Geometry check sheet. Reference: drawing and pictorial views, mm from the part's lowest x, y, z. A direction names the side the tool comes from. Give positions to 0.01 mm unless a question says otherwise; leave off trailing zeros. Write each loop counter-clockwise with the first axis right and the second up, starting at its lowest first coordinate (ties: lowest second). Pieces come first, ordered by that corner, then holes. Notation, with made-up numbers: M 78.5,52.5 L 96.5,52.5 A14 cw 96.5,72.5 Z; hole C -34,10.5 d7. An arc over 180 degrees is marked long. Write item = value, one per line. Start each with the question number.
1) Cross-section at B-B, the plane z = 29.5. Record the cut outline in (x, y).
2) Scan lines: line 1 along X through (y, z) = (6.25, 6); line 2 along Y through (x, z) = (37, 29.1); line 3 along Z through (x, y) = (20, 4.75). Record each from-to range of solid material in increasing order. Write a range as [from, to].
3) Cross-section at C-C, the plane y = 12.5. Record the cut outline in (x, z).
4) Cross-section at D-D, the plane z = 6. Record the cut outline in (x, y), plus the area to 3 significant figures.
5) Mould release check, pull along Z, two halves, no side actions. Record for the marked faces 1, 2, 3 and 4: released by +Z, released by -Z, zero draft, split by the parting line, or undercut.
6) Go/stop test with flat-tipped pins: pin 1 (2.5 mm diameter, centred on y = 5.5, z = 28.5, fed in from -X); pin 2 (10.5 mm diameter, centred on x = 7, y = 11, fed in from -Z); pin 3 (1.2 mm diameter, centred on x = 5.5, z = 29, fed in from -Y); pin 4 (12 mm diameter, centred on y = 5.5, z = 25.5, fed in from +X). Record where each tip stops, or that it passes through.
7) Cross-section at A-A, the plane y = 3.5. Record the cut outline in (x, z), plus the area to 3 significant figures.
8) Access from +Z, -Z, +X, -X, +Y, -Y to the whole of each face (thin tool, end or side, straight path). Record for the marked faces 5, 6, 7, 8 and 9.
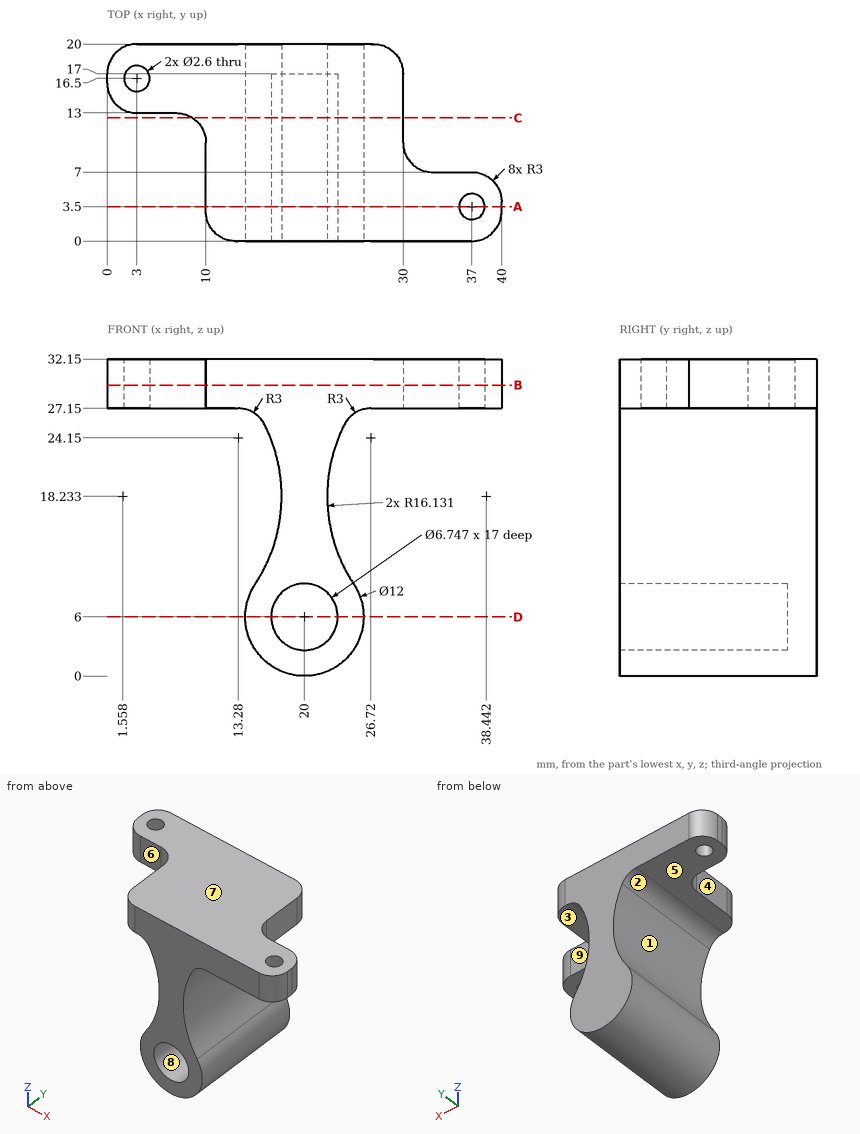
Reply:
q1.outline = M 0,16 A3 ccw 3,13 L 7,13 A3 cw 10,10 L 10,3 A3 ccw 13,0 L 37,0 A3 ccw 40,3 L 40,4 A3 ccw 37,7 L 33,7 A3 cw 30,10 L 30,17 A3 ccw 27,20 L 3,20 A3 ccw 0,17 Z; hole C 3,16.5 d2.6; hole C 37,3.5 d2.6
q2.line_1 = [14, 16.63], [23.37, 26]
q2.line_2 = [0, 2.2], [4.8, 7]
q2.line_3 = [0, 2.63], [9.37, 32.15]
q3.outline = M 8.66,27.15 L 13.28,27.15 A3 cw 15.96,25.5 A16.13 cw 15,9.32 A6 ccw long 25,9.32 A16.13 cw 24.04,25.5 A3 cw 26.72,27.15 L 30,27.15 L 30,32.15 L 8.66,32.15 Z; hole C 20,6 d6.75
q4.outline = M 14,0 L 16.63,0 L 16.63,17 L 23.37,17 L 23.37,0 L 26,0 L 26,20 L 14,20 Z
q4.area = 125 mm2
q5.face_1 = undercut
q5.face_2 = undercut
q5.face_3 = released by -Z
q5.face_4 = zero draft
q6.pin_1 = 10
q6.pin_2 = 27.15
q6.pin_3 = 13
q6.pin_4 = 40
q7.outline = M 10,27.15 L 13.28,27.15 A3 cw 15.96,25.5 A16.13 cw 15,9.32 A6 ccw long 25,9.32 A16.13 cw 24.04,25.5 A3 cw 26.72,27.15 L 35.7,27.15 L 35.7,32.15 L 10,32.15 Z; M 38.3,27.15 L 40,27.15 L 40,32.15 L 38.3,32.15 Z; hole C 20,6 d6.75
q7.area = 310 mm2
q8.face_5 = -Z, -X, +Y, -Y
q8.face_6 = +Z, -Z, -X, -Y
q8.face_7 = +Z, +X, -X, +Y, -Y
q8.face_8 = -Y
q8.face_9 = +Z, -Z, +X, +Y
